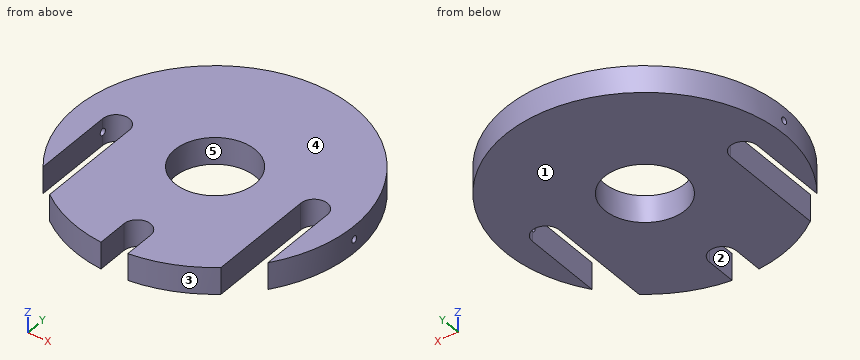
from build123d import *

# Parameters (mm, degrees)
SKETCH1_R              = 52
BOSS_EXTRUDE1_DEPTH    = 10
CUT_EXTRUDE1_DEPTH     = 10
SKETCH3_R              = 15
CUT_EXTRUDE2_DEPTH     = 10
M3_TAPPED_HOLE3_REACH  = 118.705
M3_TAPPED_HOLE3_BORE_R = 1.25


with BuildPart() as part:
    # Sketch1 → Boss-Extrude1 (new body)
    with BuildSketch(Plane.XY):
        Circle(SKETCH1_R)
    extrude(amount=BOSS_EXTRUDE1_DEPTH)

    # Sketch2 → Cut-Extrude1 (cut)
    with BuildSketch(Plane.XY.offset(10)):
        with BuildLine():
            Line((32, 0), (32, -45))
            Line((32, -45), (42, -45))
            Line((42, -45), (42, 3.54e-07))
            ThreePointArc((42, 3.54e-07), (36.999999823, 5), (32, 0))
        make_face()
        with BuildLine():
            Line((-5, -39.999999646), (-5, -55))
            Line((-5, -55), (5, -55))
            Line((5, -55), (5, -40))
            ThreePointArc((5, -40), (1.77e-07, -35), (-5, -39.999999646))
        make_face()
        with BuildLine():
            Line((-32, -45), (-42, -45))
            Line((-42, -45), (-42, 3.54e-07))
            ThreePointArc((-42, 3.54e-07), (-36.999999823, 5), (-32, 0))
            Line((-32, 0), (-32, -45))
        make_face()
    extrude(amount=-CUT_EXTRUDE1_DEPTH, mode=Mode.SUBTRACT)

    # Sketch3 → Cut-Extrude2 (cut)
    with BuildSketch(Plane.XY.offset(10)):
        Circle(SKETCH3_R)
    extrude(amount=-CUT_EXTRUDE2_DEPTH, mode=Mode.SUBTRACT)

    # M3 Tapped Hole3 bore → M3 Tapped Hole3 (cut, up to next)
    with BuildSketch(Plane(origin=(52, 0, 0), x_dir=(0, 0, -1), z_dir=(1, 0, 0)), mode=Mode.PRIVATE) as m3_tapped_hole3_sk1:
        with Locations((-5, 1e-08)):
            Circle(M3_TAPPED_HOLE3_BORE_R)
    m3_tapped_hole3_tool1 = extrude(m3_tapped_hole3_sk1.sketch, amount=-M3_TAPPED_HOLE3_REACH, mode=Mode.PRIVATE) & part.part
    m3_tapped_hole3 = m3_tapped_hole3_tool1.solids().sort_by_distance((52, 0, 5))[0]
    add(m3_tapped_hole3, mode=Mode.SUBTRACT)

    # Mirror1: M3 Tapped Hole3 across plane
    add(m3_tapped_hole3.mirror(Plane(origin=(0, 0, 0), x_dir=(0, 0, 1), z_dir=(1, 0, 0))), mode=Mode.SUBTRACT)


solid = part.part
Geometry: final body of the model. Coordinates: model frame, mm. Face numbers are marked on the shaded views. A direction names the side the tool comes from. Coordinates: 2 decimals unless noted, no trailing zeros. Loops run counter-clockwise (first coordinate to the right, second up) from the corner with the lowest first, then second, coordinate; pieces in that order, holes last. Notation, with made-up numbers: M -5,28.5 L 45,28.5 A28 ccw 45,55.5 Z; hole C 39,53.5 d5. An arc over 180 degrees is marked long. One line per item, written item: value. Start each with the question number.
1) Cut plane C-C (y = 8). Return loops of the section in (x, z), then the cut area to 3 significant figures.
2) Cut plane B-B (z = 5). Return loops of the section in (x, y).
3) Draft query along X for the marked faces 3, 4 and 5. Return one class per face: released by +X, released by -X, zero draft, split by the parting line, or undercut.
4) Material intervals for L1, parallel to X at y = -8, z = 3; L2, parallel to X at y = -21.5, z = 7.25; L3, parallel to X at y = -27, z = 1.75, sorted ascending. Write a range as from..to.
5) Pin query (flat end, axial travel): P1, Ø3, axis at y = -18.5, z = 6.5, coming from the -X side; P2, Ø3, axis at x = -15, z = 8, coming from the +Y side; P3, Ø1, axis at y = -22.5, z = 2.5, coming from the -X side; P4, Ø12, axis at x = 35.5, y = 28, coming from the -Z side. Return the tip coordinate at first contact, or that it passes through.
6) Cut plane D-D (y = -11). Return loops of the section in (x, z).
7) Cut plane A-A (x = 12.5). Return loops of the section in (y, z), then the cut area to 3 significant figures.
8) Reachability of the marked faces 1 and 2 from +Z, -Z, +X, -X, +Y, -Y: full face, straight path, thin tool, end or side. Return the list, or none.
Evaluation:
1. outline: M -51.38,0 L -12.69,0 L -12.69,10 L -51.38,10 Z; M 12.69,0 L 51.38,0 L 51.38,10 L 12.69,10 Z
1. area: 774 mm^2
2. outline: M -51.98,-1.25 A52 ccw -42,-30.66 L -42,-1.25 Z; M -51.98,1.25 L -41.84,1.25 A5 cw -32,0 L -32,-40.99 A52 ccw -5,-51.76 L -5,-40 A5 cw 5,-40 L 5,-51.76 A52 ccw 32,-40.99 L 32,0 A5 cw 41.84,1.25 L 51.98,1.25 A52 ccw Z; M 42,-30.66 A52 ccw 51.98,-1.25 L 42,-1.25 Z; hole C 0,0 d30
3. face 3: released by +X
3. face 4: zero draft
3. face 5: undercut
4. L1: -51.38..-42, -32..-12.69, 12.69..32, 42..51.38
4. L2: -47.35..-42, -32..32, 42..47.35
4. L3: -44.44..-42, -32..32, 42..44.44
5. P1: x = -49.14
5. P2: y = 50.22
5. P3: x = -47.12
5. P4: z = 0
6. outline: M -50.82,0 L -42,0 L -42,10 L -50.82,10 Z; M -32,0 L -10.2,0 L -10.2,10 L -32,10 Z; M 10.2,0 L 32,0 L 32,10 L 10.2,10 Z; M 42,0 L 50.82,0 L 50.82,10 L 42,10 Z
7. outline: M -50.48,0 L -8.29,0 L -8.29,10 L -50.48,10 Z; M 8.29,0 L 50.48,0 L 50.48,10 L 8.29,10 Z
7. area: 844 mm^2
8. face 1: -Z, +X, -X, +Y, -Y
8. face 2: +Z, -Z, -Y
